Could you check a few things on this drawing? It's one solid part, dimensions in mm from its lowest x, y, z. Coordinates: 2 decimals unless noted, no trailing zeros. Order: outer loops, then holes, each group sorted by start corner. A loop starts at its lowest first (then second) coordinate and runs counter-clockwise, first axis right, second up. Notation, with made-up numbers: (-27.75, 64.5) - (-3.75, 64.5) arc R24 ccw to (-3.75, 74.5) - close; hole circle Ø9 at (-22, -31). An arc over 180 degrees is marked (long way). Return JSON: item names as keys, results as strings. Group by question number.
1) Imagine slicing it at A-A (x = 31). Write out the boundary of the cut face in (y, z).
2) Imagine slicing it at C-C (y = 30). Give the number of separate pieces and of enclosed holes in the cut face, and give its area (3 significant figures).
3) If we mould it in two halves opening along Y, with no side actions, what happens to the marked faces 1 and 2? For each: pulls with the +Y half, pulls with the -Y half, needs draft (parallel to the pull), parting line crosses it, or undercut.
4) Imagine slicing it at B-B (z = 1.1). Write out the boundary of the cut face in (x, y).
5) For pin 1 Ø3.5 at (x, y) = (6, 31) entering from +Z, with a flat end and sliding along its axis, tell me the tip position at first contact or that it passes through.
6) If I drill on line 1 along Y through (x, z) = (6, 1.3); line 2 along Y through (x, z) = (31, 3.1); line 3 along Y through (x, z) = (52, 1.7), over which ranges is the centre line in solid material (lowest first)?
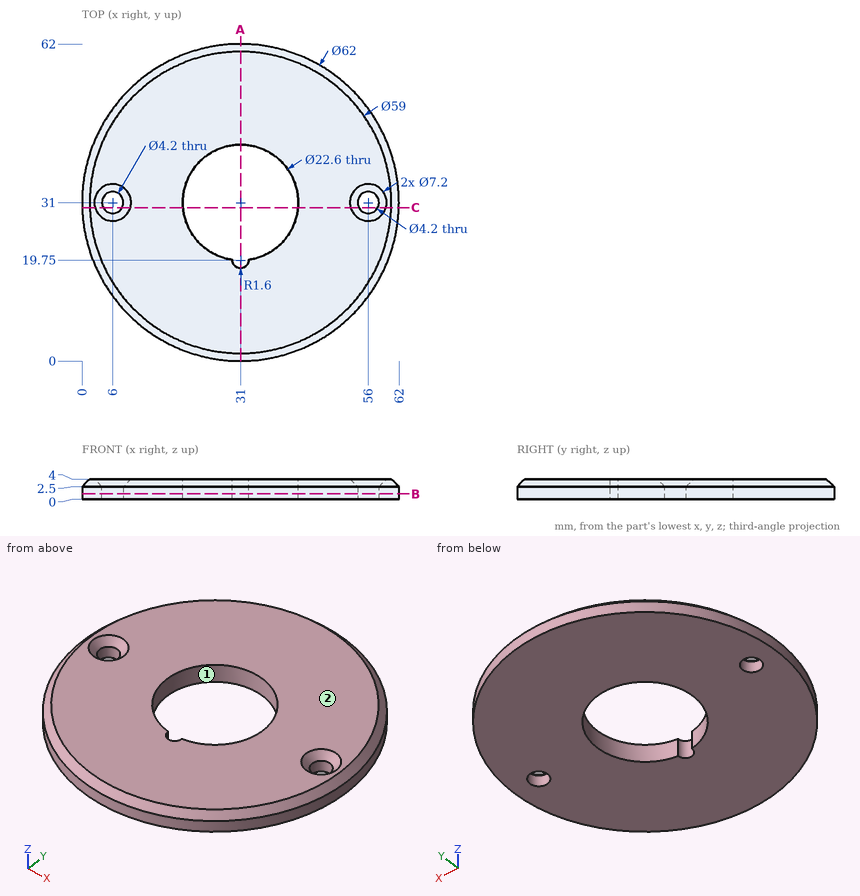
Calculated:
{
 "1": {"outline": "(0, 0) - (18.15, 0) - (18.15, 4) - (1.5, 4) - (0, 2.5) - close; (42.3, 0) - (62, 0) - (62, 2.5) - (60.5, 4) - (42.3, 4) - close"},
 "2": {"separate pieces": "4", "enclosed holes": "0", "area": "121 mm2"},
 "3": {"face 1": "undercut", "face 2": "needs draft"},
 "4": {"outline": "circle Ø62 at (31, 31); hole circle Ø4.2 at (6, 31); hole (29.4, 19.81) arc R1.6 ccw (long way) to (32.6, 19.81) arc R11.3 ccw (long way) to start; hole circle Ø4.2 at (56, 31)"},
 "5": {"pin 1": "through"},
 "6": {"line 1": "12.67 to 28.9, 33.1 to 49.33", "line 2": "0.6 to 18.15, 42.3 to 61.4", "line 3": "8.2 to 53.8"}
}
